from build123d import *

# Parameters (mm, degrees)
FILLET1_R           = 11
FILLET2_R           = 1
BOSS_EXTRUDE1_DEPTH = 10.425
CHAMFER1_SIZE       = 0.35


with BuildPart() as part:
    # Sketch1 → Revolve1 (revolve)
    with BuildSketch(Plane.XY, mode=Mode.PRIVATE) as revolve1_sk:
        with BuildLine():
            Line((0, 0), (8.5, 0))
            Line((8.5, 0), (8.5, 1))
            Line((8.5, 1), (4, 8))
            Line((4, 8), (4, 23))
            Line((4, 23), (3.5, 24))
            Line((3.5, 24), (2.5, 24))
            add(Edge.make_bspline(
                [(2.5, 24), (1.3, 23.5), (0, 23.5)],
                knots=[0, 0, 0, 1, 1, 1], degree=2))
            Line((0, 23.5), (0, 0))
        make_face()
    revolve(revolve1_sk.sketch.rotate(Axis((0, 23.5, 0), (0, -1, 0)), 180), axis=Axis((0, 23.5, 0), (0, -1, 0)))

    # Fillet1
    fillet1_edges = [part.edges().sort_by_distance(p)[0] for p in [
        (4, 8, 0),
    ]]
    fillet(fillet1_edges, radius=FILLET1_R)

    # Fillet2
    fillet2_edges = [part.edges().sort_by_distance(p)[0] for p in [
        (2.5, 24, 0),
        (3.5, 24, 0),
        (4, 23, 0),
        (8.5, 1, 0),
    ]]
    fillet(fillet2_edges, radius=FILLET2_R)

    # Sketch3 → Cut-Revolve1 (revolve, cut)
    with BuildSketch(Plane.XY, mode=Mode.PRIVATE) as cut_revolve1_sk:
        Polygon((0, 0), (3.875, 0), (3.875, 6.5), (3.05, 7.325), (3.05, 17.75), (0, 17.75), align=None)
    revolve(cut_revolve1_sk.sketch.rotate(Axis((0, 17.75, 0), (0, -1, 0)), 180), axis=Axis((0, 17.75, 0), (0, -1, 0)), mode=Mode.SUBTRACT)

    # Sketch4 → Boss-Extrude1 (add)
    with BuildSketch(Plane.XZ.offset(-17.75)):
        with BuildLine():
            Line((-2.655654345, 1.5), (2.655654345, 1.5))
            ThreePointArc((2.655654345, 1.5), (0, 3.05), (-2.655654345, 1.5))
        make_face()
        with BuildLine():
            ThreePointArc((-0.099986562, -3.048360656), (0, -3.05), (0.099986562, -3.048360656))
            ThreePointArc((0.099986562, -3.048360656), (0, -2.95), (-0.099986562, -3.048360656))
        make_face()
    extrude(amount=BOSS_EXTRUDE1_DEPTH)

    # Chamfer1
    # the kernel refuses this chamfer: 0.35 mm, written as the material it takes off along each edge
    with BuildSketch(Plane(origin=(-3.555743391, 7.325, 1.5), x_dir=(0, -0.02749587661058614, 0.9996219169112968), z_dir=(1, 0, 0))) as chamfer1_piece_1_section:
        Polygon((CHAMFER1_SIZE * 0.999621916911, -CHAMFER1_SIZE * 0.0274958766106), (-CHAMFER1_SIZE * 0.0274958766106, -CHAMFER1_SIZE * 0.999621916911), (0, 0), align=None)
    chamfer1_piece_1 = extrude(amount=7.111486782, mode=Mode.PRIVATE)
    chamfer1_piece_1 = chamfer1_piece_1 & Plane(origin=(0, 7.499624527, 0), x_dir=(-1, 0, 0), z_dir=(0, 1, 0)) * Cylinder(3.05, 16, mode=Mode.PRIVATE)
    add(chamfer1_piece_1, mode=Mode.SUBTRACT)


solid = part.part
The model under review builds one solid part; all positions refer to its coordinate system, in mm. A direction names the side the tool comes from. Round coordinates to 2 decimals unless told otherwise and drop trailing zeros. Write each loop counter-clockwise with the first axis right and the second up, starting at its lowest first coordinate (ties: lowest second). Pieces come first, ordered by that corner, then holes. Notation, with made-up numbers: M -4.75,50 L 29.25,50 A23 ccw 29.25,89 Z; hole C 1,23 d1. An arc over 180 degrees is marked long. Use a Markdown table: item, result. Add a question column.
Q1. Insertion check: pin 1 (2.5 mm diameter, centred on x = -0.5, y = 13.5, fed in from -Z); pin 2 (2 mm diameter, centred on x = 1, y = 13.5, fed in from +Z); pin 3 (1.3 mm diameter, centred on x = 0, z = 2, fed in from -Y) (3 decimals). Each pin has a flat end and moves straight along its axis. Give the tip position at first contact, or say it passes through.
Q2. To check wall thickness, follow line 1 (Z direction, x = 0, y = 1.5) (3 decimals); line 2 (X direction, y = 8.5, z = -1); line 3 (Z direction, x = 0, y = 2.25) (3 decimals). State the ranges of each line that lie inside material, in increasing order.
Q3. We need section A-A, the plane y = 15. State the section outline as (x, z) points.
Q4. We need section B-B, the plane y = 19.75. State the section outline as (x, z) points.
Q5. We need section C-C, the plane y = 3.75. State the section outline as (x, z) points (3 decimals), plus the area to 3 significant figures.
Q6. The part is to be moulded in two halves that separate along X. For faces 1 (the face through (-3.695, 17.078, 1.532)), 2 (the face through (0, 17.75, 0)), 3 (the face through (4, 0, 2)), say which applies: pulls with the +X half, pulls with the -X half, needs draft (parallel to the pull), parting line crosses it, or undercut.
Q7. Machinability: for faces 4 (the face through (0.504, 3.296, -3.842)), 5 (the face through (1.27, 5.09, 5.73)), which of the approach directions +Z, -Z, +X, -X, +Y, -Y give a long, thin tool a straight path to every point of the face, cutting with its end or side? Answer none if there is none.
Findings below:
| question | item | result |
|---|---|---|
| 1 | pin 1 | stops at z = -4 |
| 1 | pin 2 | stops at z = 4 |
| 1 | pin 3 | stops at y = 7.325 |
| 2 | line 1 | z = -8.179 to -3.875, 3.875 to 8.179 |
| 2 | line 2 | x = -4.23 to -2.88, 2.88 to 4.23 |
| 2 | line 3 | z = -7.696 to -3.875, 3.875 to 7.696 |
| 3 | outline | C 0,0 d8; hole M -2.66,1.5 A3.05 ccw -0.1,-3.05 A0.1 cw 0.1,-3.05 A3.05 ccw 2.66,1.5 Z |
| 4 | outline | C 0,0 d8 |
| 5 | outline | C 0,0 d13.464; hole C 0,0 d7.75 |
| 5 | area | 95.2 mm² |
| 6 | face 1 | parting line crosses it |
| 6 | face 2 | undercut |
| 6 | face 3 | needs draft |
| 7 | face 4 | -Y |
| 7 | face 5 | +Y |
